from build123d import *

# Parameters (mm, degrees)
F0_R     = 17
F1_DEPTH = 2
F2_R     = 2
F3_DEPTH = 4
F4_R     = 0.25
F5_DEPTH = 0.2
F6_R     = 1.5
F7_DEPTH = 0.4


with BuildPart() as f1:
    # F0 (on Front) → F1 (new body, symmetric)
    with BuildSketch(Plane.XZ):
        Circle(F0_R)
    extrude(amount=F1_DEPTH, both=True)

    # F2 (on face) → F3 (cut)
    with BuildSketch(Plane.XZ.offset(2)):
        with Locations((-6.778185, 6.778185)):
            Circle(F2_R)
        with Locations((-9.5858, 0)):
            Circle(F2_R)
        with Locations((-6.778185, -6.778185)):
            Circle(F2_R)
        with Locations((0, -9.5858)):
            Circle(F2_R)
        with Locations((6.778185, -6.778185)):
            Circle(F2_R)
        with Locations((9.5858, 0)):
            Circle(F2_R)
        with Locations((6.778185, 6.778185)):
            Circle(F2_R)
        with Locations((0, 9.5858)):
            Circle(F2_R)
    extrude(amount=-F3_DEPTH, mode=Mode.SUBTRACT)

    # F4 (on face) → F5 (join)
    with BuildSketch(Plane.XZ.offset(2)):
        with Locations((-2.741827, 0.890874)):
            Circle(F4_R)
        with Locations((-2.741827, -0.890874)):
            Circle(F4_R)
        with Locations((-1.694542, -2.332337)):
            Circle(F4_R)
        with Locations((0, -2.882927)):
            Circle(F4_R)
        with Locations((1.694542, -2.332337)):
            Circle(F4_R)
        with Locations((2.741827, -0.890874)):
            Circle(F4_R)
        with Locations((2.741827, 0.890874)):
            Circle(F4_R)
        with Locations((1.694542, 2.332337)):
            Circle(F4_R)
        with Locations((0, 2.882927)):
            Circle(F4_R)
        with Locations((-1.694542, 2.332337)):
            Circle(F4_R)
    extrude(amount=F5_DEPTH)

    # F6 (on face) → F7 (join)
    with BuildSketch(Plane.XZ.offset(2)):
        Circle(F6_R)
    extrude(amount=F7_DEPTH)


solid = f1.part
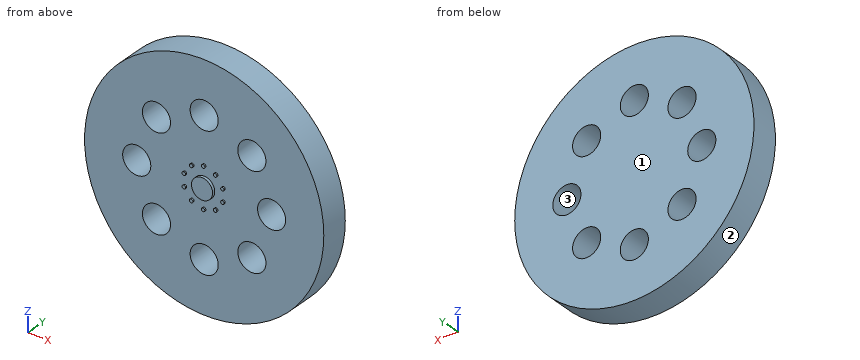
Source: CAD feature listing. Evaluate the final solid. Frame: model axes, mm. Face numbers are marked on the shaded views. Coordinates: 2 decimals unless noted, no trailing zeros. Loops run counter-clockwise (first coordinate to the right, second up) from the corner with the lowest first, then second, coordinate; pieces in that order, holes last. Notation, with made-up numbers: (26, -4.75) -> (63, -4.75) arc R20 ccw to (63, 7.25) -> close; hole circle Ø3 at (25, 31.25). An arc over 180 degrees is marked (long way). Answer in a Markdown table with one row per item. Add a question column.
Q1. Section B-B on x = 9.5. Return the cut outline in (y, z).
Q2. Section A-A on z = 0. Return the cut outline in (x, y), and give its area (3 significant figures).
Q3. Pull-direction query (X, two-part tool) for the marked faces 1, 2 and 3; classes: pulls with the +X half, pulls with the -X half, needs draft (parallel to the pull), parting line crosses it, or undercut.
Q4. Section D-D on y = -0.6. Give the number of separate pieces and of enclosed holes in the cut face, and give its area (3 significant figures).
Q5. Ray query, line 1 along X through (y, z) = (0.45, 1); line 2 along X through (y, z) = (0.75, -6.5); line 3 along X through (y, z) = (1, 8.5). Return the intervals inside material, ascending.
Q6. Section C-C on z = -11. Return the cut outline in (x, y), and give its area (3 significant figures).
Q7. Contact query for flat-ended pins moving along their axis: pin 1 Ø1 at (y, z) = (-0.5, -7) entering from -X; pin 2 Ø4.5 at (x, z) = (6.78, -6.78) entering from -Y; pin 3 Ø1 at (x, y) = (12, 0) entering from +Z. Output: stop coordinate, or through.
Computed values:
| question | item | result |
|---|---|---|
| 1 | outline | (-2, -14.1) -> (2, -14.1) -> (2, -2) -> (-2, -2) -> close; (-2, 2) -> (2, 2) -> (2, 14.1) -> (-2, 14.1) -> close |
| 2 | outline | (-17, -2) -> (-11.59, -2) -> (-11.59, 2) -> (-17, 2) -> close; (-7.59, -2) -> (-1.5, -2) -> (-1.5, -2.4) -> (1.5, -2.4) -> (1.5, -2) -> (7.59, -2) -> (7.59, 2) -> (-7.59, 2) -> close; (11.59, -2) -> (17, -2) -> (17, 2) -> (11.59, 2) -> close |
| 2 | area | 105 mm^2 |
| 3 | face 1 | needs draft |
| 3 | face 2 | parting line crosses it |
| 3 | face 3 | undercut |
| 4 | separate pieces | 1 |
| 4 | enclosed holes | 8 |
| 4 | area | 807 mm^2 |
| 5 | line 1 | x = -16.97 to -11.32, -7.85 to 7.85, 11.32 to 16.97 |
| 5 | line 2 | x = -15.71 to -8.76, -4.8 to 4.8, 8.76 to 15.71 |
| 5 | line 3 | x = -14.72 to -7.8, -5.76 to -1.68, 1.68 to 5.76, 7.8 to 14.72 |
| 6 | outline | (-12.96, -2) -> (-1.41, -2) -> (-1.41, 2) -> (-12.96, 2) -> close; (1.41, -2) -> (12.96, -2) -> (12.96, 2) -> (1.41, 2) -> close |
| 6 | area | 92.4 mm^2 |
| 7 | pin 1 | stops at x = -15.71 |
| 7 | pin 2 | stops at y = -2 |
| 7 | pin 3 | stops at z = 12.52 |
